from build123d import *

# Parameters (mm, degrees)
SKETCH_1_W                   = 130
SKETCH_1_H                   = 35
EXTRUDE_1_DEPTH              = 10
SKETCH_2_R                   = 9.5
CUT_EXTRUDE_1_DEPTH          = 5
SKETCH_3_R                   = 6
CUT_EXTRUDE_2_DEPTH          = 135.721935853
FILLET_1_R                   = 10
SKETCH_4_W                   = 80
SKETCH_4_H                   = 35
EXTRUDE_2_DEPTH              = 1.5
HOLE_WIZARD_M6_1_D           = 7
HOLE_WIZARD_M6_1_CBORE_D     = 11
HOLE_WIZARD_M6_1_CBORE_DEPTH = 6


with BuildPart() as part:
    # 草图1 → 凸台-拉伸1 (new body)
    with BuildSketch(Plane.XY):
        with Locations((65, 17.5)):
            Rectangle(SKETCH_1_W, SKETCH_1_H)
    extrude(amount=EXTRUDE_1_DEPTH)

    # 草图2 → 切除-拉伸1 (cut)
    with BuildSketch(Plane.XY.offset(10)):
        with Locations((15, 17.5)):
            Circle(SKETCH_2_R)
    extrude(amount=-CUT_EXTRUDE_1_DEPTH, mode=Mode.SUBTRACT)

    # 草图3 → 切除-拉伸2 (cut, through all)
    with BuildSketch(Plane.XY.offset(5)):
        with Locations((15, 17.5)):
            Circle(SKETCH_3_R)
    extrude(amount=-CUT_EXTRUDE_2_DEPTH, mode=Mode.SUBTRACT)

    # 圆角1
    fillet_1_edges = [part.edges().sort_by_distance(p)[0] for p in [
        (0, 35, 5),
        (0, 0, 5),
    ]]
    fillet(fillet_1_edges, radius=FILLET_1_R)

    # 草图4 → 凸台-拉伸2 (add)
    with BuildSketch(Plane.XY.offset(10)):
        with Locations((90, 17.5)):
            Rectangle(SKETCH_4_W, SKETCH_4_H)
    extrude(amount=EXTRUDE_2_DEPTH)

    # M6 六角凹头螺钉的柱形沉头孔1 (through all)
    with Locations(Plane(origin=(0, 0, 0), x_dir=(-1, 0, 0), z_dir=(0, 0, -1))):
        with Locations((-115, 11.5), (-115, 27.5), (-55, 27.5), (-55, 11.5)):
            CounterBoreHole(HOLE_WIZARD_M6_1_D / 2, HOLE_WIZARD_M6_1_CBORE_D / 2, HOLE_WIZARD_M6_1_CBORE_DEPTH)


solid = part.part
Input: part model. Units: mm. Frame: model coordinates. A direction names the side the tool comes from. Round coordinates to 2 decimals unless told otherwise and drop trailing zeros. Write each loop counter-clockwise with the first axis right and the second up, starting at its lowest first coordinate (ties: lowest second). Pieces come first, ordered by that corner, then holes.
1) Cut plane A-A (x = 115). Return the cut outline in (y, z).
2) Ray query, L1, parallel to Y at x = 115, z = 3.8; L2, parallel to Y at x = 115, z = 8.2; L3, parallel to X at y = 28, z = 8. Return the intervals inside material, ascending.
3) Draft query along Y for faces 4 (the cylindrical face through (2.85, 3.01, 5.07)), 5 (the flat face through (64, 18, 0)), 6 (the flat face through (15, 11, 5)). Return one class per face: pulls with the +Y half, pulls with the -Y half, needs draft (parallel to the pull), parting line crosses it, or undercut.
4) Contact query for flat-ended pins moving along their axis: P1, Ø17.5, axis at x = 37, y = 20, coming from the +Z side; P2, Ø9, axis at x = 55, y = 11.5, coming from the -Z side; P3, Ø1.2, axis at y = 16, z = 11, coming from the -X side. Output: stop coordinate, or through.
5) Reachability of faces 1 (the cylindrical face through (51.503, 11.654, 8.788)), 2 (the cylindrical face through (7.46, 11.72, 7.54)), 3 (the flat face through (111, 28, 6)) from +Z, -Z, +X, -X, +Y, -Y: full face, straight path, thin tool, end or side. Return the list, or none.
6) Cut plane C-C (y = 29). Return the cut outline in (x, z), then the cut area to 3 significant figures.
7) Cut plane B-B (z = 7.5). Return the cut outline in (x, y), then the cut area to 3 significant figures.
8) Cut plane D-D (x = 15). Return the cut outline in (y, z), then the cut area to 3 significant figures.
Geometry says:
1. outline: (0, 0) - (6, 0) - (6, 6) - (8, 6) - (8, 11.5) - (0, 11.5) - close; (15, 6) - (17, 6) - (17, 0) - (22, 0) - (22, 6) - (24, 6) - (24, 11.5) - (15, 11.5) - close; (31, 6) - (33, 6) - (33, 0) - (35, 0) - (35, 11.5) - (31, 11.5) - close
2. L1: y = 0 to 6, 17 to 22, 33 to 35
2. L2: y = 0 to 8, 15 to 24, 31 to 35
2. L3: x = 0.46 to 51.54, 58.46 to 111.54, 118.46 to 130
3. face 4: pulls with the -Y half
3. face 5: needs draft
3. face 6: undercut
4. P1: stops at z = 10
4. P2: stops at z = 6
4. P3: stops at x = 50
5. face 1: +Z, -Z
5. face 2: +Z
5. face 3: -Z
6. outline: (0.83, 0) - (49.71, 0) - (49.71, 6) - (51.84, 6) - (51.84, 11.5) - (50, 11.5) - (50, 10) - (0.83, 10) - close; (58.16, 6) - (60.29, 6) - (60.29, 0) - (109.71, 0) - (109.71, 6) - (111.84, 6) - (111.84, 11.5) - (58.16, 11.5) - close; (118.16, 6) - (120.29, 6) - (120.29, 0) - (130, 0) - (130, 11.5) - (118.16, 11.5) - close
6. area: 1,220 mm2
7. outline: (0, 10) arc R10 ccw to (10, 0) - (130, 0) - (130, 35) - (10, 35) arc R10 ccw to (0, 25) - close; hole circle Ø19 at (15, 17.5); hole circle Ø7 at (55, 11.5); hole circle Ø7 at (55, 27.5); hole circle Ø7 at (115, 11.5); hole circle Ø7 at (115, 27.5)
7. area: 4,070 mm2
8. outline: (0, 0) - (11.5, 0) - (11.5, 5) - (8, 5) - (8, 10) - (0, 10) - close; (23.5, 0) - (35, 0) - (35, 10) - (27, 10) - (27, 5) - (23.5, 5) - close
8. area: 195 mm2
